Design review of the part built by this model. Coordinates are the model's own, in mm. Coordinates: 2 decimals unless noted, no trailing zeros. Loops run counter-clockwise (first coordinate to the right, second up) from the corner with the lowest first, then second, coordinate; pieces in that order, holes last. Notation, with made-up numbers: (42, -32) -> (67, -32) arc R13 cw to (67, -7) -> close; hole circle Ø1 at (-15.75, 27.25). An arc over 180 degrees is marked (long way). Use CSV: the item, a comma, the result in double quotes.
Autodesk Inventor part; units mm, degrees
ref_plane "YZ Plane" through (0, 0, 0) normal (1, 0, 0) x (0, 1, 0)
ref_plane "XZ Plane" through (0, 0, 0) normal (0, 1, 0) x (-1, 0, 0)
ref_plane "XY Plane" through (0, 0, 0) normal (0, 0, 1) x (1, 0, 0)
sketch "Эскиз1" plane through (0, 0, 0) normal (0, 1, 0) x (-1, 0, 0)
  circle A0 centre (0, 0) radius 13.5
  dimension "d0" = 27
extrude "Выдавливание1" add sketch "Эскиз1" along normal blind 6
sketch "Эскиз2" plane through (0, 6, 0) normal (0, 1, 0) x (1, 0, 0)
  circle A0 centre (0, 0) radius 6
  dimension "d3" = 12
extrude "Выдавливание2" add sketch "Эскиз2" along normal blind 19
sketch "Эскиз3" plane through (0, 25, 0) normal (0, 1, 0) x (1, 0, 0)
  circle A0 centre (0, 0) radius 4
  dimension "d6" = 8
extrude "Выдавливание3" cut sketch "Эскиз3" against normal through all
chamfer "Фаска1" distance 0.25 angle 45 5 edges at (-4, 25, 0) (-6, 25, 0) (13.5, 6, 0) (13.5, 0, 0) (-4, 0, 0)
sketch "Эскиз4" plane through (0, 6, 0) normal (0, 1, 0) x (1, 0, 0)
  circle A0 centre (0, -10.5) radius 1.5
  circle A1 centre (-10.5, 0) radius 1.5
  circle A2 centre (0, 10.5) radius 1.5
  circle A3 centre (10.5, 0) radius 1.5
  dimension "d13" = 3
  dimension "d14" = 3
  dimension "d15" = 3
  dimension "d16" = 3
extrude "Выдавливание4" cut sketch "Эскиз4" against normal through all
chamfer "Фаска2" distance 0.25 angle 45 8 edges at (-12, 6, 0) (-1.5, 6, -10.5) (9, 6, 0) (-1.5, 6, 10.5) (-1.5, 0, 10.5) (-12, 0, 0) (9, 0, 0) (-1.5, 0, -10.5)
thread "Резьба1"
properties part number "Tin-bronze M8 nut for Z- axis"
Item 1: Add section A-A (z = 0). State how many separate pieces and enclosed holes the cut face has, then the cut area to 3 significant figures.
Checked values:
separate pieces,"4"
enclosed holes,"0"
area,"153 mm^2"
Item 2: To check wall thickness, follow line 1 along X through (y, z) = (10.75, 0); line 2 along Z through (x, y) = (0, 1.65); line 3 along Z through (x, y) = (0.25, 12). State the ranges of each line that lie inside material, in increasing order.
Checked values:
line 1,"-6 to -4, 4 to 6"
line 2,"-13.5 to -12, -9 to -4, 4 to 9, 12 to 13.5"
line 3,"-5.99 to -3.99, 3.99 to 5.99"
Item 3: Add section D-D (y = 6.75). Give the boundary of the cut face in (x, z), then the cut area to 3 significant figures.
Checked values:
outline,"circle Ø12 at (0, 0); hole circle Ø8 at (0, 0)"
area,"62.8 mm^2"
Item 4: Clearance check with flat-ended pins moving along their axes: pin 1 (4 mm diameter, centred on x = -1, y = 18.5, fed in from -Z); pin 2 (1.5 mm diameter, centred on x = 3, z = -1.5, fed in from +Y); pin 3 (2 mm diameter, centred on x = 8, y = 4, fed in from +Z). State where each tip first meets the part, or that it passes through.
Checked values:
pin 1,"z = -6"
pin 2,"y = 24.85"
pin 3,"z = 11.54"
Item 5: Draft analysis for pull direction X (two halves, no side actions). For faces 1 (the face through (-6, 6, -3)), 2 (the face through (-6, 15, 0)), 3 (the face through (-0.867, 12.672, 3.905)), state which applies: pulls with the +X half, pulls with the -X half, needs draft (parallel to the pull), parting line crosses it, or undercut.
Checked values:
face 1,"needs draft"
face 2,"parting line crosses it"
face 3,"undercut"
Item 6: Add section B-B (y = 4). Give the boundary of the cut face in (x, z).
Checked values:
outline,"circle Ø27 at (0, 0); hole circle Ø3 at (-10.5, 0); hole circle Ø8 at (0, 0); hole circle Ø3 at (0, -10.5); hole circle Ø3 at (0, 10.5); hole circle Ø3 at (10.5, 0)"
